from build123d import *

# Parameters (mm, degrees)
SKETCH1_W           = 100
SKETCH1_H           = 100
BOSS_EXTRUDE1_DEPTH = 150
SKETCH2_W           = 1.709615385
SKETCH2_H           = 19.05
CUT_EXTRUDE1_DEPTH  = 30


with BuildPart() as part:
    # Sketch1 → Boss-Extrude1 (new body)
    with BuildSketch(Plane.XY):
        with Locations((-5.555555556, 7.828282828)):
            Rectangle(SKETCH1_W, SKETCH1_H)
    extrude(amount=BOSS_EXTRUDE1_DEPTH)

    # Sketch2 → Cut-Extrude1 (cut)
    with BuildSketch(Plane(origin=(44.444444444, 0, 0), x_dir=(0, 0, -1), z_dir=(1, 0, 0))):
        Polygon((-116.409832449, 17.921320019), (-114.646791584, 17.921320019), (-110.914640142, 3.939108481), (-105.373654565, 17.921320019), (-105.12560769, 17.921320019), (-99.680024757, 4.045959442), (-95.932608892, 17.921320019), (-94.184832449, 17.921320019), (-99.321310815, -1.128679981), (-99.565541584, -1.128679981), (-105.297332449, 13.433579635), (-111.090181007, -1.128679981), (-111.338227882, -1.128679981), align=None)
        with Locations((-89.910793987, 8.396320019)):
            Rectangle(SKETCH2_W, SKETCH2_H)
        Polygon((-84.171370911, -1.128679981), (-84.171370911, 17.921320019), (-83.812656969, 17.921320019), (-71.227140142, 2.927840452), (-71.227140142, 17.921320019), (-69.517524757, 17.921320019), (-69.517524757, -1.128679981), (-69.906767545, -1.128679981), (-82.461755526, 13.830454635), (-82.461755526, -1.128679981), align=None)
        with BuildLine():
            Line((-47.048293988, 14.425767135), (-48.544207449, 13.280935404))
            add(Edge.make_bspline(
                [(-48.544207449, 13.280935404), (-48.650919499, 13.40811304), (-48.862904888, 13.660753681), (-49.203949976, 14.01551663), (-49.559377489, 14.347886125), (-49.929051563, 14.659445498), (-50.3196262, 14.939299609), (-50.721639975, 15.202032326), (-51.141817907, 15.437532443), (-51.722852348, 15.723080981), (-52.482935637, 16.021056482), (-53.439761832, 16.270901213), (-54.438586526, 16.429947897), (-55.120019175, 16.447173677), (-55.466623315, 16.455935404)],
                knots=[0, 0, 0, 0, 0.757959112, 1.505699292, 2.245454638, 2.979532153, 3.711538275, 4.438200793, 5.171680507, 5.909471876, 7.393775596, 8.890124382, 10.418191784, 12, 12, 12, 12], degree=3))
            add(Edge.make_bspline(
                [(-55.466623315, 16.455935404), (-55.657576701, 16.453736694), (-56.037711246, 16.449359679), (-56.601855081, 16.391615726), (-57.155464688, 16.31045614), (-57.698179954, 16.190031167), (-58.229310057, 16.037780197), (-58.752327274, 15.855850444), (-59.259659252, 15.630761959), (-59.758324235, 15.38197843), (-60.23609394, 15.100977623), (-60.6881507, 14.794472094), (-61.112845783, 14.465891726), (-61.510515143, 14.11400499), (-61.881565319, 13.740396605), (-62.223307682, 13.341084974), (-62.534559701, 12.917346716), (-62.821490937, 12.474769454), (-63.0784631, 12.014642331), (-63.293618587, 11.535262305), (-63.484146466, 11.044838544), (-63.634909487, 10.537830083), (-63.7542415, 10.017804458), (-63.83657921, 9.483366026), (-63.89366646, 8.935631284), (-63.898021709, 8.56437774), (-63.900217065, 8.377239491)],
                knots=[0, 0, 0, 0, 1.054917814, 2.100044995, 3.131103042, 4.146048494, 5.169673617, 6.183595914, 7.203665975, 8.234915748, 9.262203917, 10.264457458, 11.251630812, 12.227803204, 13.197192746, 14.159520551, 15.12972552, 16.100847026, 17.073214652, 18.039054194, 19.002613845, 19.979014051, 20.95965708, 21.949030935, 22.966165397, 24, 24, 24, 24], degree=3))
            add(Edge.make_bspline(
                [(-63.900217065, 8.377239491), (-63.893349164, 8.095673306), (-63.879864952, 7.542855452), (-63.759859019, 6.733118271), (-63.577495594, 5.957398604), (-63.304179382, 5.220545462), (-62.967162836, 4.513472828), (-62.541310364, 3.848144211), (-62.048097497, 3.214505482), (-61.480546728, 2.627531723), (-60.857852215, 2.09133559), (-60.189752868, 1.619164568), (-59.477912673, 1.225564993), (-58.7301913, 0.898035913), (-57.94083488, 0.646267152), (-57.111262884, 0.46902528), (-56.243279596, 0.353407126), (-55.650174719, 0.342338052), (-55.348324036, 0.336704635)],
                knots=[0, 0, 0, 0, 1.029171465, 2.020641659, 2.987623507, 3.938342917, 4.889210282, 5.84687017, 6.821220943, 7.821438502, 8.827599549, 9.822697543, 10.807740252, 11.797342354, 12.80366471, 13.83203677, 14.896651826, 16, 16, 16, 16], degree=3))
            add(Edge.make_bspline(
                [(-55.348324036, 0.336704635), (-55.015750829, 0.345896422), (-54.361167199, 0.363988057), (-53.401221227, 0.517254827), (-52.482272274, 0.765764352), (-51.60427091, 1.113551615), (-50.769692336, 1.56566411), (-49.977230513, 2.113748271), (-49.226216536, 2.763017625), (-48.7746157, 3.258770081), (-48.544207449, 3.511704635)],
                knots=[0, 0, 0, 0, 1.028121516, 2.023589091, 2.998037872, 3.967518031, 4.937445131, 5.927275754, 6.942489185, 8, 8, 8, 8], degree=3))
            Line((-48.544207449, 3.511704635), (-47.048293988, 2.378321221))
            add(Edge.make_bspline(
                [(-47.048293988, 2.378321221), (-47.1686797, 2.222990504), (-47.408874484, 1.913073096), (-47.797810262, 1.476165647), (-48.207533838, 1.065207968), (-48.641088488, 0.683513344), (-49.093486754, 0.323444039), (-49.572851768, -0.004770214), (-50.072881788, -0.305710599), (-50.591882595, -0.581265717), (-51.129302759, -0.825743875), (-51.684498326, -1.03504224), (-52.255076173, -1.215336282), (-52.841062383, -1.36366468), (-53.443672431, -1.479440151), (-54.060731725, -1.55683581), (-54.693572046, -1.609859658), (-55.120517495, -1.614692457), (-55.336875719, -1.617141519)],
                knots=[0, 0, 0, 0, 0.986787822, 1.968848986, 2.935600012, 3.899624008, 4.868462664, 5.837806735, 6.815139263, 7.798259679, 8.787526145, 9.778297419, 10.776456485, 11.791383307, 12.812564526, 13.85620153, 14.913611965, 16, 16, 16, 16], degree=3))
            add(Edge.make_bspline(
                [(-55.336875719, -1.617141519), (-55.541764821, -1.615715531), (-55.946907648, -1.612895816), (-56.545070853, -1.567218448), (-57.127399857, -1.504899166), (-57.692230321, -1.411063595), (-58.242644557, -1.300332259), (-58.773652881, -1.151898705), (-59.290480526, -0.985623955), (-59.791051066, -0.790198241), (-60.275790289, -0.569674448), (-60.743134748, -0.320437534), (-61.192869502, -0.044583385), (-61.629416149, 0.251807457), (-62.046325855, 0.578255343), (-62.447211471, 0.930226597), (-62.834320949, 1.306534912), (-63.073821277, 1.577887757), (-63.194237497, 1.714318817)],
                knots=[0, 0, 0, 0, 1.114604814, 2.203992996, 3.262667896, 4.300477797, 5.318619304, 6.316056647, 7.298880507, 8.271930387, 9.238335007, 10.195173496, 11.151986948, 12.108099108, 13.064862484, 14.031167946, 15.010108607, 16, 16, 16, 16], degree=3))
            add(Edge.make_bspline(
                [(-63.194237497, 1.714318817), (-63.387108643, 1.951307289), (-63.770522424, 2.422423098), (-64.261063644, 3.185979653), (-64.680966766, 3.98318519), (-65.020469992, 4.818227945), (-65.285878583, 5.689234153), (-65.469744801, 6.596642881), (-65.589224249, 7.539606681), (-65.602887392, 8.180975488), (-65.609832449, 8.506987087)],
                knots=[0, 0, 0, 0, 0.994628077, 1.977248131, 2.950237994, 3.925870899, 4.908910175, 5.911660606, 6.938484602, 8, 8, 8, 8], degree=3))
            add(Edge.make_bspline(
                [(-65.609832449, 8.506987087), (-65.601367753, 8.849644627), (-65.584713991, 9.523801945), (-65.44322259, 10.513171605), (-65.215608857, 11.46105279), (-64.892320077, 12.365676028), (-64.482443808, 13.231799411), (-63.976113238, 14.05280654), (-63.37921065, 14.833947978), (-62.69641746, 15.563371124), (-61.947658107, 16.230335315), (-61.145822848, 16.817109081), (-60.292481108, 17.305428704), (-59.397033944, 17.713622102), (-58.452776163, 18.02737268), (-57.461722397, 18.247009311), (-56.425734875, 18.383718186), (-55.718912244, 18.401000389), (-55.359772353, 18.409781558)],
                knots=[0, 0, 0, 0, 1.032925535, 2.032216505, 3.007276963, 3.968222605, 4.92396291, 5.891752235, 6.871517503, 7.883894988, 8.900124299, 9.891468569, 10.874487609, 11.85992873, 12.854644235, 13.869047385, 14.917252991, 16, 16, 16, 16], degree=3))
            add(Edge.make_bspline(
                [(-55.359772353, 18.409781558), (-55.140890727, 18.407157349), (-54.707636592, 18.401962991), (-54.066725727, 18.351310988), (-53.442743919, 18.266872646), (-52.835261288, 18.151940895), (-52.241322477, 18.009298188), (-51.66546688, 17.823477421), (-51.104315456, 17.611007158), (-50.561407284, 17.36630465), (-50.039347204, 17.091621386), (-49.538297813, 16.790002064), (-49.062239082, 16.461820608), (-48.607821207, 16.109868182), (-48.18264583, 15.726698881), (-47.774641211, 15.322851966), (-47.397663057, 14.886695008), (-47.164963524, 14.579691011), (-47.048293988, 14.425767135)],
                knots=[0, 0, 0, 0, 1.096760587, 2.17092713, 3.219439832, 4.250915756, 5.268269357, 6.278326846, 7.281116186, 8.274029601, 9.260640565, 10.235837813, 11.203064059, 12.156899882, 13.114053108, 14.069676657, 15.032185724, 16, 16, 16, 16], degree=3))
        make_face()
        Polygon((-43.14060168, 17.921320019), (-41.430986295, 17.921320019), (-41.430986295, 10.105935404), (-31.661755526, 10.105935404), (-31.661755526, 17.921320019), (-29.952140142, 17.921320019), (-29.952140142, -1.128679981), (-31.661755526, -1.128679981), (-31.661755526, 8.15208925), (-41.430986295, 8.15208925), (-41.430986295, -1.128679981), (-43.14060168, -1.128679981), align=None)
    extrude(amount=-CUT_EXTRUDE1_DEPTH, mode=Mode.SUBTRACT)


solid = part.part
Input: part model. Units: mm. Frame: model coordinates. A direction names the side the tool comes from. Give positions to 0.01 mm unless a question says otherwise; leave off trailing zeros. Write item = value, one per line. Start each with the question number.
1) Reachability of faces 4 (the flat face through (44.444, 7, 74)), 5 (the flat face through (14.444, 10, 107)) from +Z, -Z, +X, -X, +Y, -Y: full face, straight path, thin tool, end or side. Return the list, or none.
2) Draft query along Y for faces 1 (the flat face through (-6, 9, 150)), 2 (the flat face through (-6, -42.172, 74)), 3 (the flat face through (29.65, 10.53, 77.61)). Return one class per face: +Y half, -Y half, draft (parallel to the pull), parting line (faces both ways), or undercut.
3) Material intervals for line 1 along Y through (x, z) = (20, 61.5), sorted ascending. Write a range as [from, to].
4) Cut plane A-A on x = 34. Count the separate pieces of the cut face and the enclosed holes in it, then the cut area to 3 significant figures.
Solved:
q1.face_4 = +Z, -Z, +X, +Y, -Y
q1.face_5 = +X
q2.face_1 = draft
q2.face_2 = -Y half
q2.face_3 = undercut
q3.line_1 = [-42.17, 0.17], [2.66, 14.12], [16.55, 57.83]
q4.separate_pieces = 1
q4.enclosed_holes = 5
q4.area = 14,600 mm2
